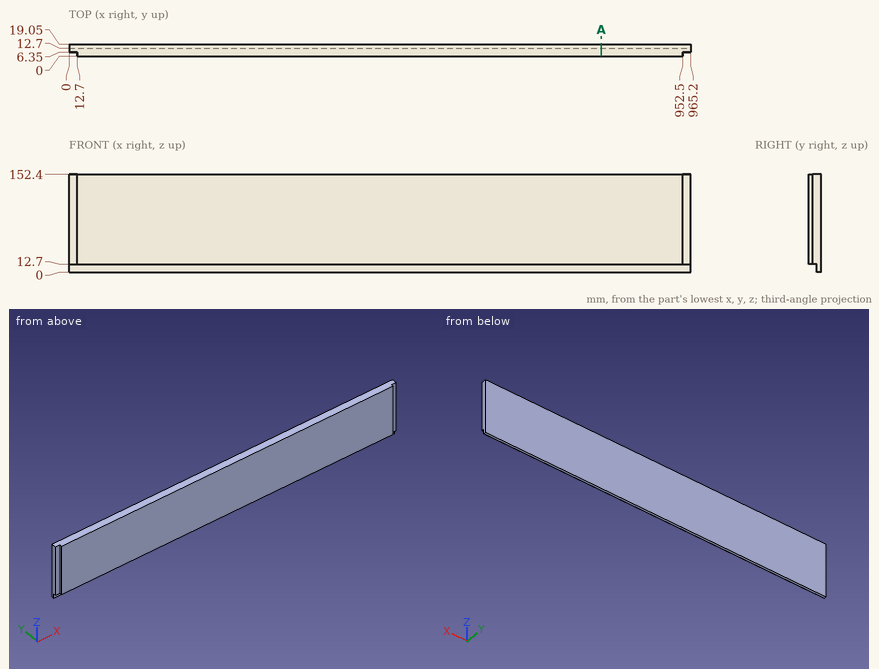
Design review of the part shown in the three views and the two pictorial views. Dimensions are in mm from the part's minimum x, y and z. Round coordinates to 2 decimals unless told otherwise and drop trailing zeros. Order: outer loops, then holes, each group sorted by start corner. A loop starts at its lowest first (then second) coordinate and runs counter-clockwise, first axis right, second up.
(1) Take a section at A-A, the plane x = 826.5. State the section outline as (y, z) points.
Working result:
outline: (0, 12.7) - (12.7, 12.7) - (12.7, 0) - (19.05, 0) - (19.05, 152.4) - (0, 152.4) - close
(2) For P1, Ø2, axis at x = 730.5, y = 5.5, coming from the -Z side; P2, Ø4, axis at x = 270, z = 5.5, coming from the -Y side; P3, Ø5, axis at x = 371, y = 11.5, coming from the -Z side; P4, Ø10, axis at x = 959, z = 84, coming from the -Y side, all flat-tipped, find the tip position at first contact; note any pin that passes through.
Working result:
P1: stops at z = 12.7
P2: stops at y = 12.7
P3: stops at z = 0
P4: stops at y = 6.35
(3) Wall thickness on L1, parallel to Z at x = 820, y = 7.5; L2, parallel to X at y = 1.25, z = 79: over which ranges is each line inside the solid? List them lowest first.
Working result:
L1: z = 12.7 to 152.4
L2: x = 12.7 to 952.5
